Geometry: final body of the model. Coordinates: model frame, mm. Face numbers are marked on the shaded views. A direction names the side the tool comes from. Round coordinates to 2 decimals unless told otherwise and drop trailing zeros. Loops run counter-clockwise (first coordinate to the right, second up) from the corner with the lowest first, then second, coordinate; pieces in that order, holes last. Notation, with made-up numbers: (52.5, -32.75) - (84.5, -32.75) arc R23 cw to (84.5, 2.25) - close; hole circle Ø11 at (-32.5, 68). An arc over 180 degrees is marked (long way). Answer as CSV lines item,"result".
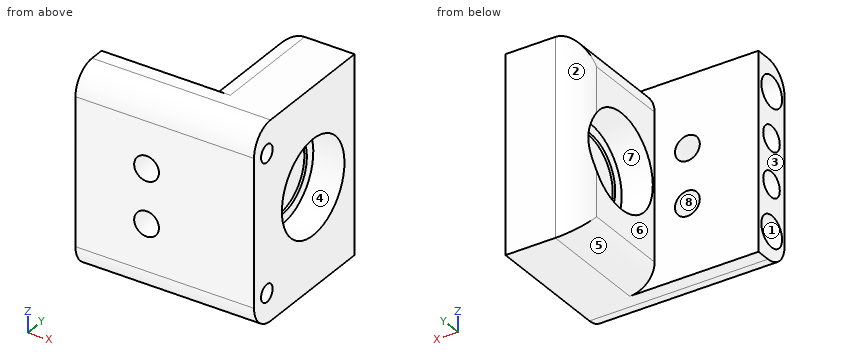
from build123d import *

# Parameters (mm, degrees)
BOSS_EXTRUDE1_DEPTH                            = 20
SKETCH2_R                                      = 1.27
CUT_EXTRUDE1_DEPTH                             = 4.000000128
SKETCH3_R                                      = 4.8006
CUT_EXTRUDE2_DEPTH                             = 3.175
SKETCH4_R                                      = 3.81
CUT_EXTRUDE3_DEPTH                             = 0.254
CUT_EXTRUDE4_START                             = -3.175
SKETCH5_R                                      = 4.8006
CUT_EXTRUDE4_DEPTH                             = 3.175
CUT_EXTRUDE5_START                             = -0.254
SKETCH6_R                                      = 3.81
CUT_EXTRUDE5_DEPTH                             = 0.254
CBORE_FOR_0_SOCKET_HEAD_CAP_SCREW1_D           = 1.778
CBORE_FOR_0_SOCKET_HEAD_CAP_SCREW1_CBORE_D     = 3.175
CBORE_FOR_0_SOCKET_HEAD_CAP_SCREW1_CBORE_DEPTH = 14.732
FILLET1_R                                      = 2.54
SKETCH10_R                                     = 1.2635
CUT_EXTRUDE6_DEPTH                             = 77.059452864


with BuildPart() as part:
    # Sketch1 → Boss-Extrude1 (new body)
    with BuildSketch(Plane.XY):
        Polygon((-71.742285041, 0), (-71.742285041, -4), (-53.530479711, -4), (-53.530479711, 11.43), (-61.150490131, 11.43), (-61.150490131, 0), align=None)
    extrude(amount=-BOSS_EXTRUDE1_DEPTH)

    # Sketch2 → Cut-Extrude1 (cut)
    with BuildSketch(Plane.ZY.offset(71.742285041)):
        with Locations((-12.286, -2)):
            Circle(SKETCH2_R)
        with Locations(Location((-7.714, -2, 0), (0, 0, 180))):
            Circle(SKETCH2_R)
    extrude(amount=-CUT_EXTRUDE1_DEPTH, mode=Mode.SUBTRACT)

    # Sketch3 → Cut-Extrude2 (cut)
    with BuildSketch(Plane.ZY.offset(61.150490131)):
        with Locations((-10, 5.08)):
            Circle(SKETCH3_R)
    extrude(amount=-CUT_EXTRUDE2_DEPTH, mode=Mode.SUBTRACT)

    # Sketch4 → Cut-Extrude3 (cut)
    with BuildSketch(Plane.ZY.offset(57.975490131)):
        with Locations((-10, 5.08)):
            Circle(SKETCH4_R)
    extrude(amount=-CUT_EXTRUDE3_DEPTH, mode=Mode.SUBTRACT)

    # Sketch5 → Cut-Extrude4 (cut)
    with BuildSketch(Plane(origin=(-53.530479711, 0, 0), x_dir=(0, 0, -1), z_dir=(1, 0, 0)).offset(CUT_EXTRUDE4_START)):
        with Locations(Location((10, 5.08, 0), (0, 0, 180))):
            Circle(SKETCH5_R)
    extrude(amount=CUT_EXTRUDE4_DEPTH, mode=Mode.SUBTRACT)

    # Sketch6 → Cut-Extrude5 (cut)
    with BuildSketch(Plane(origin=(-56.705479711, 0, 0), x_dir=(0, 0, -1), z_dir=(1, 0, 0)).offset(CUT_EXTRUDE5_START)):
        with Locations(Location((10, 5.08, 0), (0, 0, 180))):
            Circle(SKETCH6_R)
    extrude(amount=CUT_EXTRUDE5_DEPTH, mode=Mode.SUBTRACT)

    # CBORE for #0 Socket Head Cap Screw1 (through all)
    with Locations(Plane.ZY.offset(71.742285041)):
        with Locations((-16.952, -2.032), (-3.048, -2.032)):
            CounterBoreHole(CBORE_FOR_0_SOCKET_HEAD_CAP_SCREW1_D / 2, CBORE_FOR_0_SOCKET_HEAD_CAP_SCREW1_CBORE_D / 2, CBORE_FOR_0_SOCKET_HEAD_CAP_SCREW1_CBORE_DEPTH)

    # Fillet1
    # the kernel refuses this fillet: 2.54 mm, written as the material it takes off along each edge
    with BuildSketch(Plane(origin=(-78.092285041, -4, -20), x_dir=(0, 1, 0), z_dir=(1, 0, 0))) as fillet1_piece_1:
        with BuildLine():
            CenterArc((FILLET1_R, FILLET1_R), FILLET1_R, 180, 90)
            Line((0, FILLET1_R), (0, 0))
            Line((0, 0), (FILLET1_R, 0))
        make_face()
    extrude(amount=30.91180533, mode=Mode.SUBTRACT)
    with BuildSketch(Plane(origin=(-61.150490131, 11.43, 6.35), x_dir=(0, -1, 0), z_dir=(0, 0, -1))) as fillet1_piece_2:
        with BuildLine():
            CenterArc((FILLET1_R, -FILLET1_R), FILLET1_R, 90, 90)
            Line((0, -FILLET1_R), (0, 0))
            Line((0, 0), (FILLET1_R, 0))
        make_face()
    extrude(amount=32.7, mode=Mode.SUBTRACT)
    with BuildSketch(Plane(origin=(-61.150490131, 17.78, -20), x_dir=(1, 0, 0), z_dir=(0, -1, 0))) as fillet1_piece_3:
        with BuildLine():
            CenterArc((FILLET1_R, FILLET1_R), FILLET1_R, 180, 90)
            Line((0, FILLET1_R), (0, 0))
            Line((0, 0), (FILLET1_R, 0))
        make_face()
    extrude(amount=17.78, mode=Mode.SUBTRACT)
    with BuildSketch(Plane(origin=(-61.150490131, 17.78, 0), x_dir=(1, 0, 0), z_dir=(0, -1, 0))) as fillet1_piece_4:
        with BuildLine():
            CenterArc((FILLET1_R, -FILLET1_R), FILLET1_R, 90, 90)
            Line((0, -FILLET1_R), (0, 0))
            Line((0, 0), (FILLET1_R, 0))
        make_face()
    extrude(amount=17.78, mode=Mode.SUBTRACT)
    with BuildSketch(Plane(origin=(-78.092285041, -4, 0), x_dir=(0, 1, 0), z_dir=(1, 0, 0))) as fillet1_piece_5:
        with BuildLine():
            CenterArc((FILLET1_R, -FILLET1_R), FILLET1_R, 90, 90)
            Line((0, -FILLET1_R), (0, 0))
            Line((0, 0), (FILLET1_R, 0))
        make_face()
    extrude(amount=30.91180533, mode=Mode.SUBTRACT)

    # Sketch10 → Cut-Extrude6 (cut, through all)
    with BuildSketch(Plane.XZ.offset(4)):
        with Locations((-64.492285063, -7.249999912)):
            Circle(SKETCH10_R)
        with Locations(Location((-64.492285063, -12.750000088, 0), (0, 0, 180))):
            Circle(SKETCH10_R)
    extrude(amount=-CUT_EXTRUDE6_DEPTH, mode=Mode.SUBTRACT)


solid = part.part
(1) Section B-B (x = -65.5). Output: boundary loops of the cut face in (y, z) (1 decimal).
Findings below:
outline,"(-4, -17.5) arc R2.5 ccw to (-1.5, -20) - (0, -20) - (0, -13.5) - (-4, -13.5) - close; (-4, -12) - (0, -12) - (0, -8) - (-4, -8) - close; (-4, -6.5) - (0, -6.5) - (0, 0) - (-1.5, 0) arc R2.5 ccw to (-4, -2.5) - close; hole circle Ø3.2 at (-2, -17); hole circle Ø3.2 at (-2, -3)"
(2) Section A-A (y = -1.75). Give the number of separate pieces and of enclosed holes in the cut face, and give its area (3 significant figures).
Findings below:
separate pieces,"3"
enclosed holes,"2"
area,"230 mm2"
(3) Access query for the marked faces 4, 5, 6, 7 and 8. Directions: +Z, -Z, +X, -X, +Y, -Y. A direction counts if a zero-diameter tool reaches every point of the face in a straight line with its end or side. Return the directions, or none.
Findings below:
face 4,"+X"
face 5,"-Z, -X, +Y"
face 6,"+Z, -Z, -X, +Y"
face 7,"-X"
face 8,"+Y, -Y"
(4) Pin query (flat end, axial travel): P1, Ø2, axis at y = 5, z = -7, coming from the -X side; P2, Ø2.5, axis at y = -2.032, z = -16.952, coming from the -X side; P3, Ø8.5, axis at y = 5.08, z = -10, coming from the +X side; P4, Ø1, axis at y = -2, z = -17, coming from the -X side. Return the tip coordinate at first contact, or that it passes through.
Findings below:
P1,"x = -57.98"
P2,"x = -57.01"
P3,"x = -56.71"
P4,"through"
(5) Section D-D (z = -10). Output: boundary loops of the cut face in (x, y).
Findings below:
outline,"(-71.74, -4) - (-53.53, -4) - (-53.53, 0.28) - (-56.71, 0.28) - (-56.71, 1.27) - (-56.96, 1.27) - (-56.96, 8.89) - (-56.71, 8.89) - (-56.71, 9.88) - (-53.53, 9.88) - (-53.53, 11.43) - (-58.61, 11.43) arc R2.54 ccw to (-60.95, 9.88) - (-57.98, 9.88) - (-57.98, 8.89) - (-57.72, 8.89) - (-57.72, 1.27) - (-57.98, 1.27) - (-57.98, 0.28) - (-61.15, 0.28) - (-61.15, 0) - (-71.74, 0) - close"
(6) Draft query along Y for the marked faces 1, 2 and 3. Return one class per face: pulls with the +Y half, pulls with the -Y half, needs draft (parallel to the pull), parting line crosses it, or undercut.
Findings below:
face 1,"undercut"
face 2,"pulls with the +Y half"
face 3,"needs draft"
(7) Section C-C (x = -69.75). Output: boundary loops of the cut face in (y, z) (1 decimal).
Findings below:
outline,"(-4, -17.5) arc R2.5 ccw to (-1.5, -20) - (0, -20) - (0, 0) - (-1.5, 0) arc R2.5 ccw to (-4, -2.5) - close; hole circle Ø3.2 at (-2, -17); hole circle Ø3.2 at (-2, -3); hole circle Ø2.5 at (-2, -12.3); hole circle Ø2.5 at (-2, -7.7)"
(8) Material intervals for line 1 along X through (y, z) = (-1.5, -12.75); line 2 along Y through (x, z) = (-54.8, -10); line 3 along Y through (x, z) = (-57.8, -10), sorted ascending.
Findings below:
line 1,"-67.74 to -65.76, -63.23 to -53.53"
line 2,"-4 to 0.28, 9.88 to 11.43"
line 3,"-4 to 1.27, 8.89 to 11.43"
